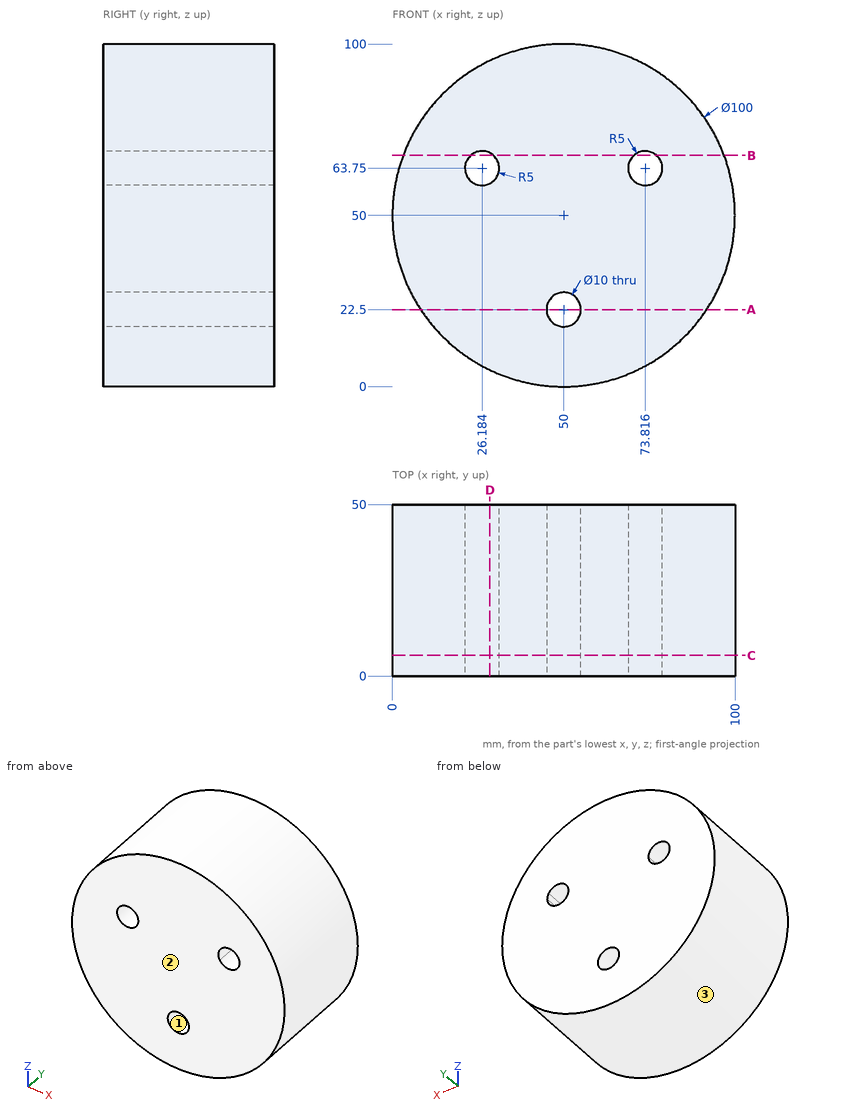
Drawing for the job (mm, zero at the part's lowest x, y, z). Give positions to 0.01 mm unless a question says otherwise; leave off trailing zeros. Loops run counter-clockwise (first coordinate to the right, second up) from the corner with the lowest first, then second, coordinate; pieces in that order, holes last.
Item 1: Slice it at B-B (z = 67.5). Write the cut outline in (x, y), plus the area to 3 significant figures.
Check values:
outline: (3.16, 0) - (22.88, 0) - (22.88, 50) - (3.16, 50) - close; (29.49, 0) - (70.51, 0) - (70.51, 50) - (29.49, 50) - close; (77.12, 0) - (96.84, 0) - (96.84, 50) - (77.12, 50) - close
area: 4,020 mm2
Item 2: Slice it at D-D (x = 28.5). Write the cut outline in (y, z), plus the area to 3 significant figures.
Check values:
outline: (0, 4.86) - (50, 4.86) - (50, 59.32) - (0, 59.32) - close; (0, 68.18) - (50, 68.18) - (50, 95.14) - (0, 95.14) - close
area: 4,070 mm2
Item 3: Drop flat-ended pins along their axis: P1, Ø6, axis at y = 37, z = 86.5, coming from the +X side; P2, Ø2, axis at y = 17, z = 78.5, coming from the +X side; P3, Ø1.5, axis at x = 18.5, y = 41.5, coming from the +Z side. Give the stop position or say it passes through.
Check values:
P1: stops at x = 87.12
P2: stops at x = 91.76
P3: stops at z = 89.43
Item 4: Mould opens along Z. For the marked faces 1, 2 and 3 say: +Z half, -Z half, draft (parallel to the pull), parting line (faces both ways), or undercut.
Check values:
face 1: undercut
face 2: draft
face 3: parting line
Item 5: Slice it at C-C (y = 6). Give the number of separate pieces and of enclosed holes in the cut face, plus the area to 3 significant figures.
Check values:
separate pieces: 1
enclosed holes: 3
area: 7,620 mm2
Item 6: Drill centre lines: line 1 along Z through (x, y) = (50, 21); line 2 along Z through (x, y) = (46.5, 18); line 3 along X through (y, z) = (12, 22) (1 decimal). Where is each one in solid material? Low to high.
Check values:
line 1: z = 0 to 17.5, 27.5 to 100
line 2: z = 0.12 to 18.93, 26.07 to 99.88
line 3: x = 8.6 to 45, 55 to 91.4
Item 7: Slice it at A-A (z = 22.5). Write the cut outline in (x, y).
Check values:
outline: (8.24, 0) - (45, 0) - (45, 50) - (8.24, 50) - close; (55, 0) - (91.76, 0) - (91.76, 50) - (55, 50) - close
